from build123d import *

# Parameters (mm, degrees)
EXTRUDE_2_DEPTH     = 5
SKETCH_2_R          = 1.5
CUT_EXTRUDE_1_DEPTH = 4
SKETCH_3_R          = 5.05
CUT_EXTRUDE_2_DEPTH = 3
CHAMFER_1_SIZE      = 0.5
FILLET_1_R          = 10
FILLET_2_R          = 2


with BuildPart() as part:
    # 草图1 → 凸台-拉伸2 (new body)
    with BuildSketch(Plane(origin=(0, 0, 0), x_dir=(0, 0, -1), z_dir=(1, 0, 0))):
        Polygon((25, 25), (25, 37.5), (28, 37.5), (28, -12.5), (25, -12.5), (25, 0), (0, 0), (0, 25), align=None)
    extrude(amount=EXTRUDE_2_DEPTH)

    # 草图2 → 切除-拉伸1 (cut)
    with BuildSketch(Plane.XY.offset(-25)):
        with Locations((2.5, 34.5)):
            Circle(SKETCH_2_R)
        with Locations((2.5, -9.5)):
            Circle(SKETCH_2_R)
    extrude(amount=-CUT_EXTRUDE_1_DEPTH, mode=Mode.SUBTRACT)

    # 草图3 → 切除-拉伸2 (cut)
    with BuildSketch(Plane.ZY):
        with Locations((-8, 12.5)):
            Circle(SKETCH_3_R)
    extrude(amount=-CUT_EXTRUDE_2_DEPTH, mode=Mode.SUBTRACT)

    # 倒角1
    chamfer_1_edges = [part.edges().sort_by_distance(p)[0] for p in [
        (0, 12.5, -13.05),
    ]]
    chamfer(chamfer_1_edges, length=CHAMFER_1_SIZE)

    # 圆角1
    fillet_1_edges = [part.edges().sort_by_distance(p)[0] for p in [
        (2.5, 25, 0),
        (2.5, 0, 0),
    ]]
    fillet(fillet_1_edges, radius=FILLET_1_R)

    # 圆角2
    fillet_2_edges = [part.edges().sort_by_distance(p)[0] for p in [
        (2.5, 25, -25),
        (2.5, 0, -25),
    ]]
    fillet(fillet_2_edges, radius=FILLET_2_R)


solid = part.part
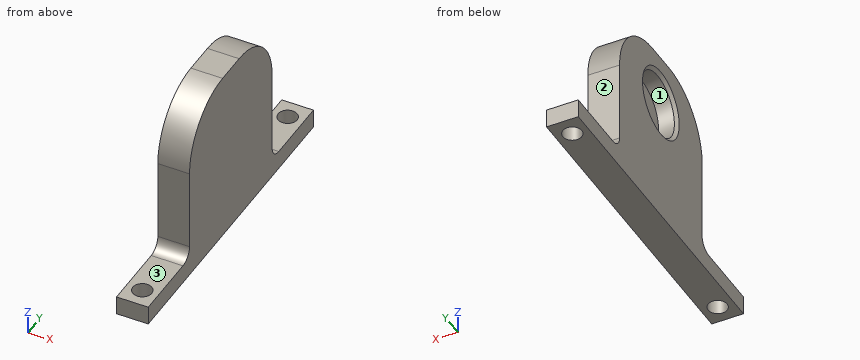
Read the model definition and answer for the solid it produces. Units are mm, in the model's axes. Face numbers are marked on the shaded views. A direction names the side the tool comes from. Coordinates: 2 decimals unless noted, no trailing zeros. Loops run counter-clockwise (first coordinate to the right, second up) from the corner with the lowest first, then second, coordinate; pieces in that order, holes last. Notation, with made-up numbers: (14, 74) - (19, 74) arc R20 ccw to (19, 85) - close; hole circle Ø10 at (77.25, -8). An arc over 180 degrees is marked (long way). Answer in a Markdown table with one row per item.
Q1. Straight lines are drawn through the part: line 1 along Y through (x, z) = (2.5, -26.6); line 2 along Y through (x, z) = (3.2, -25.5); line 3 along Y through (x, z) = (1.7, -15.25). For each, find the intervals that lie inside material, in ascending order. Write a range as [from, to].
Here are the results:
| item | result |
|---|---|
| line 1 | y = [-12.5, -11], [-8, 33], [36, 37.5] |
| line 2 | y = [-12.5, -10.83], [-8.17, 33.17], [35.83, 37.5] |
| line 3 | y = [0, 25] |
Q2. Find section A-A on x = 2.5. Write down the section's boundary in (y, z).
Here are the results:
| item | result |
|---|---|
| outline | (-12.5, -28) - (-11, -28) - (-11, -25) - (-12.5, -25) - close; (-8, -28) - (33, -28) - (33, -25) - (27, -25) arc R2 cw to (25, -23) - (25, -10) arc R10 ccw to (15, 0) - (10, 0) arc R10 ccw to (0, -10) - (0, -23) arc R2 cw to (-2, -25) - (-8, -25) - close; (36, -28) - (37.5, -28) - (37.5, -25) - (36, -25) - close; hole circle Ø10.1 at (12.5, -8) |
Q3. Find section B-B on y = 34.5. Write down the section's boundary in (x, z).
Here are the results:
| item | result |
|---|---|
| outline | (0, -28) - (1, -28) - (1, -25) - (0, -25) - close; (4, -28) - (5, -28) - (5, -25) - (4, -25) - close |
Q4. Find section D-D on z = -8. Write down the section's boundary in (x, y), plus the area to 3 significant figures.
Here are the results:
| item | result |
|---|---|
| outline | (0, 0.2) - (5, 0.2) - (5, 24.8) - (0, 24.8) - (0, 18.05) - (0.5, 17.55) - (3, 17.55) - (3, 7.45) - (0.5, 7.45) - (0, 6.95) - close |
| area | 92.4 mm^2 |
Q5. Given P1, Ø12, axis at y = 15, z = -15.5, coming from the -X side; P2, Ø3, axis at y = 13.5, z = -6.5, coming from the -X side; P3, Ø3, axis at x = 2, z = -12, coming from the -Y side; P4, Ø1, axis at x = 1, z = -6.5, coming from the -Y side, each flat-ended and moving along its own axis, determine where each tip first touches the part or whether it passes through.
Here are the results:
| item | result |
|---|---|
| P1 | stops at x = 0 |
| P2 | stops at x = 3 |
| P3 | stops at y = 0 |
| P4 | stops at y = 0.46 |
Q6. For the marked faces 1, 2 and 3, determine the directions among +Z, -Z, +X, -X, +Y, -Y from which every point of the face is accessible in a straight line to the end or side of a thin tool.
Here are the results:
| item | result |
|---|---|
| face 1 | -X |
| face 2 | +Z, +X, -X, +Y |
| face 3 | +Z, +X, -X, -Y |
Q7. Find section C-C on y = 12.5. Write down the section's boundary in (x, z).
Here are the results:
| item | result |
|---|---|
| outline | (0, -28) - (5, -28) - (5, 0) - (0, 0) - (0, -2.45) - (0.5, -2.95) - (3, -2.95) - (3, -13.05) - (0.5, -13.05) - (0, -13.55) - close |
